Autodesk Fusion 360 part; units mm, degrees
sketch "Sketch1" plane through (0, 0, 0) normal (0, 0, 1) x (1, 0, 0)
  line L0 (30, -25) -> (-30, -25)
  line L1 (-30, -25) -> (-30, 25)
  line L2 (-30, 25) -> (30, 25)
  line L3 (30, 25) -> (30, -25)
  line L4 (30, -25) -> (-30, 25) construction
  line L5 (-30, -25) -> (30, 25) construction
  line L6 (-30, -25) -> (-27.147, -22.1964)
  line L7 (-30, -25) -> (-34, -25) construction
  circle A0 centre (-27.147, -22.1964) radius 1.115
  circle A1 centre (-27.147, -22.1964) radius 2.5
  line L8 (-29.6396, 25) -> (-26.7866, 22.1964)
  line L9 (-29.6396, 25) -> (-25.6396, 25) construction
  circle A2 centre (-26.7866, 22.1964) radius 1.115
  circle A3 centre (-26.7866, 22.1964) radius 2.5
  line L10 (30, 25) -> (27.0005, 22.0005)
  line L11 (30, 25) -> (25.758, 25) construction
  circle A4 centre (27.0005, 22.0005) radius 1.115
  circle A5 centre (27.0005, 22.0005) radius 2.5
  line L12 (30, -25) -> (30, -35)
  line L13 (30, -35) -> (40, -35)
  line L14 (40, -35) -> (-40, -35)
  line L15 (-40, -35) -> (-40, 35)
  line L16 (-40, 35) -> (40, 35)
  line L17 (40, 35) -> (40, -35)
  dimension "d1" = 60
  dimension "d2" = 50
  dimension "d3" = 135.5
  dimension "d4" = 4
  dimension "d5" = 2.23
  dimension "d6" = 5
  dimension "d7" = 44.5
  dimension "d8" = 4
  dimension "d9" = 2.23
  dimension "d10" = 5
  dimension "d11" = 45
  dimension "d12" = 4.242
  dimension "d13" = 2.23
  dimension "d14" = 5
  dimension "d17" = 10
  dimension "d18" = 10
  dimension "d19" = 80
  dimension "d20" = 70
extrude "Extrude1" add sketch "Sketch1" along normal blind 10 contours A5 | A3 | A1 | L0 L1 L2 L3
extrude "Extrude2" cut 1 faces at (9.9936, -8.452, 10) along direction (0, 0, -1) blind 5
extrude "Extrude3" add sketch "Sketch1" along normal blind 24 contours L13 L14 L15 L16 L17
extrude "Extrude4" add 1 faces at (-10, 31.6667, 24) along direction (0, 0, 1) blind 2.6
extrude "Extrude5" cut 1 faces at (30, 8.3333, 12.2) along direction (1, 0, 0) blind 2.5
extrude "Extrude6" cut 1 faces at (10.8333, 25, 19.4) along direction (0, 1, 0) blind 2.5
extrude "Extrude7" cut 1 faces at (11.6667, -25, 12.2) along direction (0, -1, 0) blind 2.5
extrude "Extrude8" cut 1 faces at (-30, -8.3333, 19.4) along direction (-1, 0, 0) blind 2.5
sketch "Sketch2" plane through (0, 0, 26.6) normal (0, 0, 1) x (-1, 0, 0)
  line L0 (-32.5, 27.5) -> (32.5, 27.5)
  line L1 (32.5, 27.5) -> (32.5, -27.5)
  line L2 (32.5, -27.5) -> (-32.5, -27.5)
  line L3 (-32.5, -27.5) -> (-32.5, 27.5)
  line L4 (-40, -35) -> (40, -35)
  line L5 (40, -35) -> (40, 35)
  line L6 (40, 35) -> (-40, 35)
  line L7 (-40, 35) -> (-40, -35)
sketch "Sketch3" plane through (0, 35, 0) normal (0, 1, 0) x (-1, 0, 0)
  line L0 (-40, 0) -> (40, 0)
  line L1 (40, 0) -> (40, 26.6)
  line L2 (40, 26.6) -> (-40, 26.6)
  line L3 (-40, 26.6) -> (-40, 0)
  line L4 (40, 10.1) -> (14.2, 10.1)
  line L5 (14.2, 26.6) -> (14.2, 10.1)
  line L6 (21.7, 15.1) -> (6.7, 15.1)
  line L7 (6.7, 15.1) -> (6.7, 5.1)
  line L8 (6.7, 5.1) -> (21.7, 5.1)
  line L9 (21.7, 5.1) -> (21.7, 15.1)
  line L10 (21.7, 15.1) -> (6.7, 5.1) construction
  line L11 (6.7, 15.1) -> (21.7, 5.1) construction
  point P0 (14.2, 10.1)
  dimension "d36" = 25.8
  dimension "d37" = 16.5
  dimension "d38" = 15
  dimension "d39" = 10
extrude "Extrude9" cut sketch "Sketch3" against normal blind 22 contours L4 L5 L6 L7 L8 L9 | L4 L5 L6 L9
extrude "Extrude10" add 1 faces at (-6.7, 32.5, 11.7667) along direction (-1, 0, 0) blind 2.2
extrude "Extrude11" add 1 faces at (-21.7, 32.5, 8.4333) along direction (1, 0, 0) blind 2.2
extrude "Extrude12" add 1 faces at (-12.4333, 32.5, 5.1) along direction (0, 0, 1) blind 2.2
extrude "Extrude13" cut sketch "Sketch2" against normal blind 5
extrude "Extrude14" cut 1 faces at (-10.8333, -27.5, 10.5333) along direction (0, -1, 0) blind 5
extrude "Extrude15" add 1 faces at (13.3333, -35, 7.2) along direction (0, -1, 0) blind 5
extrude "Extrude16" cut 1 faces at (-10.8333, -32.5, 10.5333) along direction (0, -1, 0) blind 7
extrude "Extrude17" add 1 faces at (13.3333, -40, 7.2) along direction (0, -1, 0) blind 7
extrude "Extrude18" cut 1 faces at (-37.5, 5.1667, 21.6) along direction (0, 0, -1) blind 5
sketch "Sketch4" plane through (0, 0, 0) normal (0, 0, -1) x (1, 0, 0)
  line L0 (-40, -35) -> (40, -35)
  line L1 (40, -35) -> (40, 47)
  line L2 (40, 47) -> (-40, 47)
  line L3 (-40, 47) -> (-40, -35)
  circle A0 centre (27.0005, -22.0005) radius 1.115
  circle A1 centre (-27.147, 22.1964) radius 1.115
  circle A2 centre (-26.7866, -22.1964) radius 1.115
sketch "Sketch5" plane through (0, 0, 16.6) normal (0, 0, 1) x (-1, 0, 0)
  line L0 (32.5, 39.5) -> (32.5, -27.5)
  line L1 (32.5, -27.5) -> (-32.5, -27.5)
  line L2 (-32.5, -27.5) -> (-32.5, 39.5)
  line L3 (-32.5, 39.5) -> (32.5, 39.5)
  line L4 (-40, 47) -> (-40, -35)
  line L5 (-40, -35) -> (40, -35)
  line L6 (40, -35) -> (40, 47)
  line L7 (40, 47) -> (-40, 47)
  line L8 (40, 47) -> (36.4645, 43.4645)
  line L9 (40, 47) -> (35, 47) construction
  circle A0 centre (36.4645, 43.4645) radius 1
  line L10 (-40, 47) -> (-36.4645, 43.4645)
  line L11 (-40, 47) -> (-35, 47) construction
  circle A1 centre (-36.4645, 43.4645) radius 1
  line L12 (-40, -35) -> (-36.4645, -31.4645)
  line L13 (-40, -35) -> (-35, -35) construction
  circle A2 centre (-36.4645, -31.4645) radius 1
  line L14 (40, -35) -> (36.4645, -31.4645)
  line L15 (40, -35) -> (35, -35) construction
  circle A3 centre (36.4645, -31.4645) radius 1
  dimension "d60" = 45
  dimension "d61" = 5
  dimension "d62" = 2
  dimension "d63" = 5
  dimension "d64" = 45
  dimension "d65" = 2
  dimension "d66" = 5
  dimension "d67" = 45
  dimension "d68" = 2
  dimension "d69" = 45
  dimension "d70" = 5
  dimension "d71" = 2
extrude "Extrude19" add sketch "Sketch4" along normal blind 5
extrude "Extrude20" cut sketch "Sketch5" against normal blind 20 contours A2 | A3 | A0 | A1
fillet "Fillet1" radius 3 4 edges at (40, -47, 5.8) (-40, -47, 5.8) (-40, 35, 5.8) (40, 35, 5.8)
fillet "Fillet2" radius 7.5 8 edges at (39.1213, 34.1213, -5) (40, -6, -5) (39.1213, -46.1213, -5) (0, -47, -5) (-39.1213, -46.1213, -5) (-40, -6, -5) (-39.1213, 34.1213, -5) (0, 35, -5)
equation "d23 = 17 mm + 5 mm + 2 mm"
equation "d36 = 25 mm + 0.8 mm"
equation "d37 = 15 mm + 1.5 mm"
Input: part model. Units: mm. Frame: model coordinates. A direction names the side the tool comes from. Coordinates: 2 decimals unless noted, no trailing zeros. Order: outer loops, then holes, each group sorted by start corner. A loop starts at its lowest first (then second) coordinate and runs counter-clockwise, first axis right, second up. Notation, with made-up numbers: (35, 32) - (53, 32) arc R14 cw to (53, 53) - close; hole circle Ø7 at (-12.5, 19). An arc over 180 degrees is marked (long way). Return JSON: item names as keys, results as strings.
Q1. Draft query along X for faces 4 (the flat face through (1, -47, 10)), 5 (the flat face through (40, -5, 10)), 6 (the cylindrical face through (-39.14, -46.1, 9.65)), 7 (the flat face through (-14, 31, 7.3)). Return one class per face: +X half, -X half, draft (parallel to the pull), parting line (faces both ways), or undercut.
The answers:
{"face 4": "draft", "face 5": "+X half", "face 6": "-X half", "face 7": "undercut"}
Q2. Access query for faces 1 (the flat face through (-36, 31, -3.4)), 2 (the flat face through (0, 27.5, 11)), 3 (the flat face through (-14, 31, 15.1)). Directions: +Z, -Z, +X, -X, +Y, -Y. A direction counts if a zero-diameter tool reaches every point of the face in a straight line with its end or side. Return the directions, or none.
The answers:
{"face 1": "none", "face 2": "+Z", "face 3": "+Y"}
Q3. Cut plane C-C (z = 8.75). Return loops of the section in (x, y).
The answers:
{"outline": "(-40, -44) arc R3 ccw to (-37, -47) - (37, -47) arc R3 ccw to (40, -44) - (40, 32) arc R3 ccw to (37, 35) - (-8.9, 35) - (-8.9, 27.5) - (32.5, 27.5) - (32.5, -39.5) - (-32.5, -39.5) - (-32.5, 27.5) - (-19.5, 27.5) - (-19.5, 35) - (-37, 35) arc R3 ccw to (-40, 32) - close; hole circle Ø2 at (-36.46, -43.46); hole circle Ø2 at (-36.46, 31.46); hole circle Ø2 at (36.46, -43.46); hole circle Ø2 at (36.46, 31.46)"}
Q4. Cut plane B-B (x = 27). Return loops of the section in (y, z), then the cut area to 3 significant figures.
The answers:
{"outline": "(-47, 2.5) arc R7.5 ccw to (-39.5, -5) - (20.89, -5) - (20.89, 5) - (-39.5, 5) - (-39.5, 16.6) - (-47, 16.6) - close; (23.12, -5) - (27.5, -5) arc R7.5 ccw to (35, 2.5) - (35, 16.6) - (27.5, 16.6) - (27.5, 5) - (23.12, 5) - close", "area": "948 mm2"}
Q5. Cut plane A-A (y = 5). Return loops of the section in (x, z).
The answers:
{"outline": "(-40, 2.5) arc R7.5 ccw to (-32.5, -5) - (32.5, -5) arc R7.5 ccw to (40, 2.5) - (40, 16.6) - (32.5, 16.6) - (32.5, 5) - (-32.5, 5) - (-32.5, 16.6) - (-40, 16.6) - close"}
Q6. Cut plane D-D (x = 11.5). Return loops of the section in (y, z).
The answers:
{"outline": "(-47, 2.5) arc R7.5 ccw to (-39.5, -5) - (27.5, -5) arc R7.5 ccw to (35, 2.5) - (35, 16.6) - (27.5, 16.6) - (27.5, 5) - (-39.5, 5) - (-39.5, 16.6) - (-47, 16.6) - close"}
Q7. First-contact query: pin 1 (4 mm diameter, centred on x = 21, y = -15, fed in from +Z); pin 2 (6 mm diameter, centred on x = -11.5, y = 33, fed in from -Z); pin 3 (2 mm diameter, centred on y = -28.5, z = -0.5, fed in from +X). Flat tips, straight axial feed; report the tip coordinate or a pass-through.
The answers:
{"pin 1": "stops at z = 5", "pin 2": "stops at z = -4.57", "pin 3": "stops at x = 39.73"}
Q8. Ray query, probe 1 along X at (y, z) = (10.5, 9.25); probe 2 along X at (y, z) = (30, 12.5); probe 3 along Y at (x, z) = (12, 14). Return the intervals inside material, ascending.
The answers:
{"probe 1": "x = -40 to -32.5, 32.5 to 40", "probe 2": "x = -40 to -19.5, -8.9 to 40", "probe 3": "y = -47 to -39.5, 27.5 to 35"}
